from build123d import *

# Parameters (mm, degrees)
F2_DEPTH = 11.1125
F3_W     = 76.2
F3_H     = 760.3047809925
F3_W_2   = 11.1125
F4_DEPTH = 11.1125
F5_W     = 76.2
F5_H     = 760.3047809925
F5_W_2   = 11.1125
F6_DEPTH = 11.1125


# Not quite as in the source:
# - a length typed as a fraction of an inch, garbled in the dataset ("3 / 203.2 mm" for 3/8 in), is restored


with BuildPart() as f2:
    # F1 (on face) → F2 (new body)
    with BuildSketch(Plane.YZ):
        with BuildLine():
            Line((91.1791006611, 248.0211066645), (-244.2313490084, 930.3430176805))
            ThreePointArc((-244.2313490084, 930.3430176805), (-457.2, 995.0936292205), (-507.6086509916, 778.282061482))
            Line((-507.6086509916, 778.2820614821), (-84.4057673278, 146.6471358655))
            ThreePointArc((-84.4057673278, 146.6471358655), (50.8, 115.2118189755), (91.1791006611, 248.0211066645))
        make_face()
        with BuildLine():
            ThreePointArc((-171.1045716164, 321.6783965077), (-172.951087632, 331.5040451939), (-167.114914439, 339.6214386156))
            Line((-167.114914439, 339.6214386156), (-36.3148932715, 418.5429465727))
            ThreePointArc((-36.3148932715, 418.5429465727), (-26.1769388687, 419.8548999412), (-18.3564419502, 413.2716508147))
            Line((-18.3564419502, 413.2716508147), (38.4369639182, 297.7374291963))
            ThreePointArc((38.4369639182, 297.7374291963), (39.1903819803, 288.4404814306), (33.3895763356, 281.1362682351))
            Line((33.3895763356, 281.1362682351), (-84.1895763356, 213.2519127894))
            ThreePointArc((-84.1895763356, 213.2519127894), (-93.4156133399, 211.8803743364), (-101.0902972515, 217.1813274006))
            Line((-101.0902972515, 217.1813274006), (-171.1045716164, 321.6783965077))
        make_face(mode=Mode.SUBTRACT)
        with BuildLine():
            ThreePointArc((-311.133120346, 530.6725347217), (-313.0170671845, 540.3240907704), (-307.4457804185, 548.4273341718))
            Line((-307.4457804185, 548.4273341718), (-150.2040222582, 649.4231471517))
            ThreePointArc((-150.2040222582, 649.4231471517), (-139.9349605516, 650.9722969045), (-131.9432536871, 644.3400940516))
            Line((-131.9432536871, 644.3400940516), (-75.1498478186, 528.8058724331))
            ThreePointArc((-75.1498478186, 528.8058724331), (-74.3341151725, 519.7204630371), (-79.8191746138, 512.4318275976))
            Line((-79.8191746138, 512.4318275976), (-223.8400642778, 422.4731671291))
            ThreePointArc((-223.8400642778, 422.4731671291), (-233.2289400031, 420.8264391554), (-241.1188459812, 426.1754656147))
            Line((-241.1188459812, 426.1754656147), (-311.133120346, 530.6725347217))
        make_face(mode=Mode.SUBTRACT)
        with BuildLine():
            ThreePointArc((-451.1616690757, 739.6666729358), (-453.0700486814, 749.1976530431), (-447.6800561765, 757.2865018686))
            Line((-447.6800561765, 757.2865018686), (-263.9965610234, 880.3566198713))
            ThreePointArc((-263.9965610234, 880.3566198713), (-253.6404511337, 882.0731569492), (-245.5300654239, 875.4085372884))
            Line((-245.5300654239, 875.4085372884), (-188.7366595555, 759.87431567))
            ThreePointArc((-188.7366595555, 759.87431567), (-187.8814953559, 750.930274215), (-193.1588501861, 743.6586368923))
            Line((-193.1588501861, 743.6586368923), (-363.6214768428, 631.6256714009))
            ThreePointArc((-363.6214768428, 631.6256714009), (-373.1138065223, 629.7906580687), (-381.1473947108, 635.1696038288))
            Line((-381.1473947108, 635.1696038288), (-451.1616690757, 739.6666729358))
        make_face(mode=Mode.SUBTRACT)
    extrude(amount=F2_DEPTH)

    # F3 (on face) → F4 (join)
    with BuildSketch(Plane(origin=(0, 171.626899801, 84.3670043542), x_dir=(-1, 0, 0), z_dir=(0, 0.8974320931, 0.4411526247))):
        with Locations((-49.2125, 562.5105918184)):
            Rectangle(F3_W, F3_H)
        with Locations((38.1, 562.5105918184)):
            Rectangle(F3_W, F3_H)
        with Locations((-5.55625, 562.5105918184)):
            Rectangle(F3_W_2, F3_H)
    extrude(amount=F4_DEPTH)

    # F5 (on face) → F6 (join)
    with BuildSketch(Plane(origin=(0, 9.558561252, 6.404349287), x_dir=(1, 0, 0), z_dir=(0, -0.8307654265, -0.5566226785))):
        with Locations((-38.1, 548.9639251518)):
            Rectangle(F5_W, F5_H)
        with Locations((49.2125, 548.9639251518)):
            Rectangle(F5_W, F5_H)
        with Locations((5.55625, 548.9639251518)):
            Rectangle(F5_W_2, F5_H)
    extrude(amount=F6_DEPTH)


solid = f2.part
Verification items for the finished model (mm, model axes). A direction names the side the tool comes from. Coordinates: 2 decimals unless noted, no trailing zeros. Order: outer loops, then holes, each group sorted by start corner. A loop starts at its lowest first (then second) coordinate and runs counter-clockwise, first axis right, second up.
Item 1: Section check B-B, the plane y = 0. Enter the section's corners in (x, z), then the cut area to 3 significant figures.
Filled in:
outline: (-76.2, 433.51) - (0, 433.51) - (0, 375.93) - (11.11, 375.93) - (11.11, 433.51) - (87.31, 433.51) - (87.31, 458.7) - (-76.2, 458.7) - close; (0, 101.6) - (11.11, 101.6) - (11.11, 261.86) - (0, 261.86) - close
area: 6,540 mm2
Item 2: Depth check by flat-ended pin: pin 1 (8 mm diameter, centred on x = 24.5, z = 629.5, fed in from -Y); pin 2 (1.5 mm diameter, centred on x = 29, z = 909, fed in from -Y); pin 3 (1.5 mm diameter, centred on x = -31, z = 307, fed in from -Y). Enter the tip coordinate at first touch or a pass-through.
Filled in:
pin 1: stops at y = -423.98
pin 2: stops at y = -234.11
pin 3: stops at y = -205.72
Item 3: Section check D-D, the plane y = -213.5. Enter the section's corners in (x, z), then the cut area to 3 significant figures.
Filled in:
outline: (-76.2, 319.36) - (87.31, 319.36) - (87.31, 339.32) - (11.11, 339.32) - (11.11, 428.93) - (0, 428.93) - (0, 339.32) - (-76.2, 339.32) - close; (-76.2, 867.83) - (0, 867.83) - (0, 810.25) - (11.11, 810.25) - (11.11, 867.83) - (87.31, 867.83) - (87.31, 893.02) - (-76.2, 893.02) - close; (0, 608.77) - (11.11, 608.77) - (11.11, 730.29) - (0, 730.29) - close
area: 10,400 mm2
Item 4: Release check for a two-part mould opening along Z. For faces 5 (the face through (-76.2, -69, 587)), 6 (the face through (4.4, -308.2, 460.7)), 7 (the face through (-38.63, -298.97, 466.89)) record: +Z half, -Z half, draft (parallel to the pull), parting line (faces both ways), or undercut.
Filled in:
face 5: draft
face 6: -Z half
face 7: undercut
Item 5: Section check C-C, the plane z = 399. Enter the section's corners in (x, y), then the cut area to 3 significant figures.
Filled in:
outline: (-76.2, -266.86) - (87.31, -266.86) - (87.31, -253.49) - (11.11, -253.49) - (11.11, -68.7) - (0, -68.7) - (0, -253.49) - (-76.2, -253.49) - close; (-76.2, 16.96) - (0, 16.96) - (0, -11.34) - (11.11, -11.34) - (11.11, 16.96) - (87.31, 16.96) - (87.31, 29.34) - (-76.2, 29.34) - close
area: 6,580 mm2
Item 6: Access from +Z, -Z, +X, -X, +Y, -Y to the whole of each face (thin tool, end or side, straight path). Record for faces 1 (the face through (87.312, -69, 587)), 2 (the face through (5.478, -24.577, 247.669)), 3 (the face through (49.746, -78.874, 593.958)), 4 (the face through (0, -241, 595)).
Filled in:
face 1: +Z, -Z, +X, +Y, -Y
face 2: +X, -X
face 3: +X
face 4: -X
Item 7: Section check A-A, the plane x = -22.5. Enter the section's corners in (y, z), then the cut area to 3 significant figures.
Filled in:
outline: (-516.84, 772.1) - (-93.64, 140.46) - (-84.41, 146.65) - (-507.61, 778.28) - close; (-244.23, 930.34) - (91.18, 248.02) - (101.15, 252.92) - (-234.26, 935.25) - close
area: 16,900 mm2
Item 8: Material ranges on L1, parallel to Y at x = 44, z = 643.5; L2, parallel to Y at x = 61, z = 610; L3, parallel to X at y = -154, z = 385, recorded low to high.
Filled in:
L1: y = -430.68 to -417.3, -103.23 to -90.84
L2: y = -408.23 to -394.86, -86.76 to -74.38
L3: x = 0 to 11.11
